from build123d import *

# Parameters (mm, degrees)
F0_W         = 95.7279466093
F0_H         = 73.0648599565
F1_DEPTH     = 25.4
F2_T         = -3.175
F3_W         = 36.0267900012
F3_H         = 26.902483505
F4_DEPTH     = 22.225
F6_DEPTH     = 38.1
F7_T         = 2.54
F7_T3_DEPTH  = 8.255
F7_T5_DEPTH  = 8.255
F7_T7_DEPTH  = 27.305
F7_T9_DEPTH  = 31.982483505
F7_T11_DEPTH = 41.1067900012
F7_T13_DEPTH = 58.431156608
F7_T15_DEPTH = 71.7948599565
F7_T17_DEPTH = 94.4579466093
F7_T19_DEPTH = 44.8923764515
F8_W         = 26.3507906348
F8_H         = 12.0985915035
F9_DEPTH     = 3.175
F10_W        = 21.4841477573
F10_H        = 13.7384773314
F11_DEPTH    = 3.175
F13_W        = 1.8280372024
F13_H        = 2.54
F13_W_2      = 1.4438778162
F13_W_3      = 1.4618895948
F13_W_4      = 2.1120999008
F13_W_5      = 2.54
F13_H_2      = 1.8293876201
F13_H_3      = 1.8326565623
F13_W_6      = 1.4120712876
F13_W_7      = 1.6781240702
F13_W_8      = 2.2645629942
F13_W_9      = 1.5091551468
F13_H_4      = 2.1763034165
F13_H_5      = 1.8344689161
F14_DEPTH    = 1.27
F15_DEPTH    = 2.54
F16_SIZE     = 1.27
F17_SIZE     = 1.27
F18_SIZE     = 1.27
F19_SIZE     = 1.27
F20_DEPTH    = 15.24


# Not quite as in the source:
# - a shell that OpenCascade refuses in one call is made with other operations: the cavity is built on its own and cut out


with BuildPart() as f1:
    # F0 (on Top) → F1 (new body)
    with BuildSketch(Plane.XY):
        with Locations((3.9161536843, 6.8996157497)):
            Rectangle(F0_W, F0_H)
    extrude(amount=F1_DEPTH)

    # F2
    f2_openings = [f1.faces().sort_by_distance(p)[0] for p in [
        (3.916154, 6.899616, 25.4),
    ]]
    offset(amount=F2_T, openings=f2_openings)

    # F3 (on face) → F4 (join)
    with BuildSketch(Plane.XY.offset(3.175)):
        with Locations((-22.7594246197, 26.8058039755)):
            Rectangle(F3_W, F3_H)
    extrude(amount=F4_DEPTH)

    # F5 (on face) → F6 (join)
    with BuildSketch(Plane.XY.offset(25.4)):
        Polygon((-43.9478196204, 13.354562223), (-40.7728196204, 13.354562223), (-4.7460296191, 13.354562223), (-4.7460296191, 40.257045728), (-4.7460296191, 43.432045728), (-43.9478196204, 43.432045728), align=None)
    extrude(amount=F6_DEPTH)

    # F7: shell of thickness 2.54, made by hand


with BuildPart() as f7_core1:
    # F7_t2: copy of F1
    add(f1.part)

    # the walls: a layer under each face that stays
    f7_faces = [f7_core1.faces().sort_by_distance(p)[0] for p in [
        (-43.9478196204, 31.2545690686, 52.9166666667),
        (3.9161536843, 6.8996157497, 0),
        (51.7801269889, 6.8996157497, 12.7),
        (3.9161536843, -29.6328142285, 12.7),
        (-40.7568880667, -27.1973188967, 25.4),
        (-4.7460296191, 28.3933039755, 33.3375),
        (3.9161536843, 6.8996157497, 3.175),
        (21.9295486849, 40.257045728, 14.2875),
        (48.6051269889, 6.8996157497, 14.2875),
        (3.9161536843, -26.4578142285, 14.2875),
        (-40.7728196204, -6.5516260028, 14.2875),
        (-24.3469246197, 13.354562223, 33.3375),
        (35.8254692207, 43.432045728, 10.5833333333),
    ]]
    thicken(f7_faces, amount=-F7_T, mode=Mode.SUBTRACT)

    # F7_s4 → F7_t3 (cut)
    with BuildSketch(Plane.YZ.offset(-46.4878196204)):
        Polygon((13.329162223, 25.4254), (13.354562223, 22.86), (15.894562223, 22.86), (15.894562223, 25.4), align=None)
    extrude(amount=F7_T3_DEPTH, mode=Mode.SUBTRACT)

    # F7_s6 → F7_t5 (cut)
    with BuildSketch(Plane.XZ.offset(-45.972045728)):
        Polygon((-4.7206296191, 25.4254), (-4.7460296191, 22.86), (-7.2860296191, 22.86), (-7.2860296191, 25.4), align=None)
    extrude(amount=F7_T5_DEPTH, mode=Mode.SUBTRACT)

    # F7_s8 → F7_t7 (cut)
    with BuildSketch(Plane.XY.offset(0.635)):
        Polygon((-4.7206296191, 40.231645728), (-7.2860296191, 40.257045728), (-7.2860296191, 42.797045728), (-4.7460296191, 42.797045728), align=None)
        Polygon((48.5797269889, 40.231645728), (48.6051269889, 42.797045728), (51.1451269889, 42.797045728), (51.1451269889, 40.257045728), align=None)
        Polygon((48.5797269889, -26.4324142285), (51.1451269889, -26.4578142285), (51.1451269889, -28.9978142285), (48.6051269889, -28.9978142285), align=None)
        Polygon((-40.7474196204, -26.4324142285), (-40.7728196204, -28.9978142285), (-43.3128196204, -28.9978142285), (-43.3128196204, -26.4578142285), align=None)
        Polygon((-40.7474196204, 13.329162223), (-43.3128196204, 13.354562223), (-43.3128196204, 15.894562223), (-40.7728196204, 15.894562223), align=None)
    extrude(amount=F7_T7_DEPTH, mode=Mode.SUBTRACT)

    # F7_s10 → F7_t9 (cut)
    with BuildSketch(Plane.XZ.offset(-42.797045728)):
        Polygon((-4.7206296191, 3.2004), (-7.2860296191, 3.175), (-7.2860296191, 0.635), (-4.7460296191, 0.635), align=None)
    extrude(amount=F7_T9_DEPTH, mode=Mode.SUBTRACT)

    # F7_s12 → F7_t11 (cut)
    with BuildSketch(Plane.YZ.offset(-43.3128196204)):
        Polygon((13.329162223, 3.2004), (13.354562223, 0.635), (15.894562223, 0.635), (15.894562223, 3.175), align=None)
    extrude(amount=F7_T11_DEPTH, mode=Mode.SUBTRACT)

    # F7_s14 → F7_t13 (cut)
    with BuildSketch(Plane.YZ.offset(-7.2860296191)):
        Polygon((40.231645728, 3.2004), (40.257045728, 0.635), (42.797045728, 0.635), (42.797045728, 3.175), align=None)
    extrude(amount=F7_T13_DEPTH, mode=Mode.SUBTRACT)

    # F7_s16 → F7_t15 (cut)
    with BuildSketch(Plane.XZ.offset(-42.797045728)):
        Polygon((48.5797269889, 3.2004), (48.6051269889, 0.635), (51.1451269889, 0.635), (51.1451269889, 3.175), align=None)
    extrude(amount=F7_T15_DEPTH, mode=Mode.SUBTRACT)

    # F7_s18 → F7_t17 (cut)
    with BuildSketch(Plane.YZ.offset(-43.3128196204)):
        Polygon((-26.4324142285, 3.2004), (-26.4578142285, 0.635), (-28.9978142285, 0.635), (-28.9978142285, 3.175), align=None)
    extrude(amount=F7_T17_DEPTH, mode=Mode.SUBTRACT)

    # F7_s20 → F7_t19 (cut)
    with BuildSketch(Plane.XZ.offset(-15.894562223)):
        Polygon((-40.7474196204, 3.2004), (-40.7728196204, 0.635), (-43.3128196204, 0.635), (-43.3128196204, 3.175), align=None)
    extrude(amount=F7_T19_DEPTH, mode=Mode.SUBTRACT)


with BuildPart() as f1_1:
    add(f1.part)

    # what is left inside the walls is the cavity
    f7_cavity = [f7_core1.part.solids().sort_by_distance(p)[0] for p in [
        (-24.346925, 40.866646, 43.18),
    ]]
    add(f7_cavity, mode=Mode.SUBTRACT)

    # F8 (on face) → F9 (cut)
    with BuildSketch(Plane.XZ.offset(-13.354562223)):
        with BuildLine():
            ThreePointArc((-11.1161526293, 15.2735915035), (-24.2915479466, 26.6703128698), (-37.466943264, 15.2735915035))
            Line((-37.466943264, 15.2735915035), (-11.1161526293, 15.2735915035))
        make_face()
        with Locations((-24.2915479466, 9.2242957518)):
            Rectangle(F8_W, F8_H)
    extrude(amount=-F9_DEPTH, mode=Mode.SUBTRACT)

    # F10 (on face) → F11 (cut)
    with BuildSketch(Plane.YZ.offset(-4.7460296191)):
        with BuildLine():
            Line((17.0049779117, 16.9134773314), (38.489125669, 16.9134773314))
            ThreePointArc((38.489125669, 16.9134773314), (27.7470517904, 27.65555121), (17.0049779117, 16.9134773314))
        make_face()
        with Locations((27.7470517904, 10.0442386657)):
            Rectangle(F10_W, F10_H)
    extrude(amount=-F11_DEPTH, mode=Mode.SUBTRACT)

    # F13 (on face) → F14 (cut)
    with BuildSketch(Plane.XY.offset(63.5)):
        with Locations((-38.0768813193, 14.624562223)):
            Rectangle(F13_W, F13_H)
        with Locations((-29.6358391643, 14.624562223)):
            Rectangle(F13_W_2, F13_H)
        with Locations((-11.5280598402, 14.624562223)):
            Rectangle(F13_W_3, F13_H)
        with Locations((-20.0523110107, 14.624562223)):
            Rectangle(F13_W_4, F13_H)
        with Locations((-42.6778196204, 23.0370378122)):
            Rectangle(F13_W_5, F13_H_2)
        with Locations((-42.6778196204, 36.6639345884)):
            Rectangle(F13_W_5, F13_H_3)
        with Locations((-38.3811965585, 42.162045728)):
            Rectangle(F13_W_6, F13_H)
        with Locations((-30.6867770851, 42.162045728)):
            Rectangle(F13_W_7, F13_H)
        with Locations((-20.6000227481, 42.162045728)):
            Rectangle(F13_W_8, F13_H)
        with Locations((-12.2982370667, 42.162045728)):
            Rectangle(F13_W_9, F13_H)
        with Locations((-6.0160296191, 35.6560815126)):
            Rectangle(F13_W_5, F13_H_4)
        with Locations((-6.0160296191, 23.3017643914)):
            Rectangle(F13_W_5, F13_H_5)
    extrude(amount=-F14_DEPTH, mode=Mode.SUBTRACT)

    # F15 (add): faces of the model
    f15_faces = [f1_1.faces().sort_by_distance(p)[0] for p in [
        (-6.8630827973, 16.9610565444, 63.5),
        (-6.0160296191, 29.3934643269, 63.5),
        (-7.3381229169, 40.8948611138, 63.5),
        (-16.2602779455, 42.162045728, 63.5),
        (-25.7900096476, 42.162045728, 63.5),
        (-34.6005000174, 42.162045728, 63.5),
        (-41.9877249706, 40.9763533581, 63.5),
        (-42.6778196204, 29.8496689647, 63.5),
        (-42.1422453408, 17.0655675422, 63.5),
        (-33.7603203952, 14.624562223, 63.5),
        (-25.0111306086, 14.624562223, 63.5),
        (-15.6276328489, 14.624562223, 63.5),
    ]]
    extrude(f15_faces, amount=F15_DEPTH)

    # F16
    f16_edges = [f1_1.edges().sort_by_distance(p)[0] for p in [
        (-10.797115, 14.624562, 66.04),
        (-12.259005, 14.624562, 66.04),
    ]]
    chamfer(f16_edges, length=F16_SIZE)

    # F17
    f17_edges = [f1_1.edges().sort_by_distance(p)[0] for p in [
        (-6.01603, 22.38453, 66.04),
        (-6.01603, 24.218999, 66.04),
        (-6.01603, 34.56793, 66.04),
        (-6.01603, 36.744233, 66.04),
    ]]
    chamfer(f17_edges, length=F17_SIZE)

    # F18
    f18_edges = [f1_1.edges().sort_by_distance(p)[0] for p in [
        (-11.543659, 42.162046, 66.04),
        (-13.052815, 42.162046, 66.04),
        (-19.467741, 42.162046, 66.04),
        (-21.732304, 42.162046, 66.04),
        (-39.087232, 42.162046, 66.04),
        (-37.675161, 42.162046, 66.04),
        (-31.525839, 42.162046, 66.04),
        (-29.847715, 42.162046, 66.04),
    ]]
    chamfer(f18_edges, length=F18_SIZE)

    # F19
    f19_edges = [f1_1.edges().sort_by_distance(p)[0] for p in [
        (-42.67782, 37.580263, 66.04),
        (-42.67782, 35.747606, 66.04),
        (-42.67782, 23.951732, 66.04),
        (-42.67782, 22.122344, 66.04),
        (-38.9909, 14.624562, 66.04),
        (-37.162863, 14.624562, 66.04),
        (-30.357778, 14.624562, 66.04),
        (-28.9139, 14.624562, 66.04),
        (-21.108361, 14.624562, 66.04),
        (-18.996261, 14.624562, 66.04),
    ]]
    chamfer(f19_edges, length=F19_SIZE)

    # F12 (on face) → F20 (join)
    with BuildSketch(Plane.YZ.offset(-41.4078196204)):
        Polygon((40.892045728, 2.54), (40.892045728, 7.8878998756), (15.894562223, 2.54), align=None)
    extrude(amount=F20_DEPTH)


solid = f1_1.part
For this review, take the finished solid that the model builds, in its own axes (mm). A direction names the side the tool comes from. Round coordinates to 2 decimals unless told otherwise and drop trailing zeros. Write each loop counter-clockwise with the first axis right and the second up, starting at its lowest first coordinate (ties: lowest second). Pieces come first, ordered by that corner, then holes. Notation, with made-up numbers: (-21, 61) - (30, 61) arc R19 cw to (30, 97) - close; hole circle Ø11 at (21, 17). An arc over 180 degrees is marked (long way). Use a Markdown table: item, result.
Q1. We need section B-B (x = 37.5). Give the boundary of the cut face in (y, z) (3 decimals).
Derived:
| item | result |
|---|---|
| outline | (-29.633, 0) - (43.432, 0) - (43.432, 25.4) - (40.257, 25.4) - (40.257, 3.175) - (-26.458, 3.175) - (-26.458, 25.4) - (-29.633, 25.4) - close |
Q2. We need section C-C (y = -12.5). Give the boundary of the cut face in (x, z) (3 decimals).
Derived:
| item | result |
|---|---|
| outline | (-43.948, 0) - (51.78, 0) - (51.78, 25.4) - (48.605, 25.4) - (48.605, 3.175) - (-40.773, 3.175) - (-40.773, 25.4) - (-43.948, 25.4) - close |
Q3. Wall thickness on line 1 along X through (y, z) = (20, 24); line 2 along Y through (x, z) = (6.5, 5); line 3 along X through (y, z) = (-12.5, 20): over which ranges is each line inside the solid? List them lowest first.
Derived:
| item | result |
|---|---|
| line 1 | x = -43.95 to -41.41, 48.61 to 51.78 |
| line 2 | y = -29.63 to -26.46, 40.26 to 43.43 |
| line 3 | x = -43.95 to -40.77, 48.61 to 51.78 |
Q4. Clearance check with flat-ended pins moving along their axes: pin 1 (2 mm diameter, centred on y = 42, z = 63.5, fed in from +X); pin 2 (10 mm diameter, centred on x = -5, z = 41, fed in from -Y); pin 3 (2.5 mm diameter, centred on x = -5.5, y = 36, fed in from +Z). State where each tip first meets the part, or that it passes through.
Derived:
| item | result |
|---|---|
| pin 1 | stops at x = -4.75 |
| pin 2 | stops at y = 13.35 |
| pin 3 | stops at z = 65.28 |
Q5. We need section A-A (z = 42). Give the boundary of the cut face in (x, y), plus the area to 3 significant figures.
Derived:
| item | result |
|---|---|
| outline | (-43.95, 13.35) - (-4.75, 13.35) - (-4.75, 43.43) - (-43.95, 43.43) - close; hole (-41.41, 15.89) - (-7.29, 15.89) - (-7.29, 40.89) - (-41.41, 40.89) - close |
| area | 326 mm2 |
Q6. The part is to be moulded in two halves that separate along X. For faces 4 (the flat face through (-18.996, 15, 64)), 5 (the flat face through (3, -29.633, 13)), 6 (the flat face through (-43.948, 16, 25)), say which applies: pulls with the +X half, pulls with the -X half, needs draft (parallel to the pull), parting line crosses it, or undercut.
Derived:
| item | result |
|---|---|
| face 4 | undercut |
| face 5 | needs draft |
| face 6 | pulls with the -X half |
Q7. We need section D-D (y = 29.5). Give the boundary of the cut face in (x, z) (3 decimals).
Derived:
| item | result |
|---|---|
| outline | (-43.948, 0) - (51.78, 0) - (51.78, 25.4) - (48.605, 25.4) - (48.605, 3.175) - (-7.286, 3.175) - (-7.286, 2.54) - (-26.168, 2.54) - (-26.168, 5.451) - (-41.408, 5.451) - (-41.408, 66.04) - (-43.948, 66.04) - close; (-7.286, 27.512) - (-4.746, 27.512) - (-4.746, 66.04) - (-7.286, 66.04) - close |
Q8. Machinability: for faces 1 (the flat face through (-6, 24.219, 64)), 2 (the flat face through (22, 40.257, 14)), 3 (the flat face through (-6, 22.385, 63)), which of the approach directions +Z, -Z, +X, -X, +Y, -Y give a long, thin tool a straight path to every point of the face, cutting with its end or side? Answer none if there is none.
Derived:
| item | result |
|---|---|
| face 1 | +Z, +X |
| face 2 | +Z |
| face 3 | +Z, +X, -X |
